Read the model definition and answer for the solid it produces. Units are mm, in the model's axes. A direction names the side the tool comes from. Coordinates: 2 decimals unless noted, no trailing zeros. Write each loop counter-clockwise with the first axis right and the second up, starting at its lowest first coordinate (ties: lowest second). Pieces come first, ordered by that corner, then holes.
(1) Section D-D on z = 32 is taken. Write down the section's boundary in (x, y), then the cut area to 3 significant figures.
(2) Section C-C on x = 30 is taken. Write down the section's boundary in (y, z), then the cut area to 3 significant figures.
(3) The mould has two halves that part along Z. Classify faces 4 (the cylindrical face through (55.07, 13.37, 24.68)), 5 (the flat face through (53, 0, 13)), 6 (the flat face through (21, 20, 10)): +Z half, -Z half, draft (parallel to the pull), parting line (faces both ways), or undercut.
(4) Given pin 1 (8 mm diameter, centred on x = 19, y = 22, fed in from +Z); pin 2 (10 mm diameter, centred on x = 36, z = 5.5, fed in from +Y) (3 decimals); pin 3 (5 mm diameter, centred on x = 51, z = 25, fed in from -Y); pin 4 (24 mm diameter, centred on y = 15, z = 32, fed in from -X), each flat-ended and moving along its own axis, determine where each tip first touches the part or whether it passes through.
(5) Section B-B on z = 8 is taken. Write down the section's boundary in (x, y).
(6) Section A-A on y = 15 is taken. Write down the section's boundary in (x, z), then the cut area to 3 significant figures.
(7) Which of the six approach directions +Z, -Z, +X, -X, +Y, -Y give full straight-line access (tool end or side, diameter ignored) to faces 1 (the cylindrical face through (17.47, 3.51, -1.48)), 2 (the flat face through (10, 19, 25)), 3 (the flat face through (7, 30, 13))?
(8) Find the intervals of material crossed by probe 1 along X at (y, z) = (28.5, 17); probe 2 along Y at (x, z) = (30, 6.5); probe 3 along X at (y, z) = (15, 0.75), in increasing order.
from build123d import *

# Parameters (mm, degrees)
F0_R     = 10
F1_DEPTH = 50
F2_R     = 10
F3_DEPTH = 40
F4_R     = 7.5
F5_DEPTH = 60.001
F6_R     = 17
F6_R_2   = 10
F7_DEPTH = 3


with BuildPart() as f1:
    # F0 (on Top) → F1 (new body)
    with BuildSketch(Plane.XY):
        with BuildLine():
            Line((43.2287565553, 0), (16.7712434447, 0))
            ThreePointArc((16.7712434447, 0), (30, -5), (43.2287565553, 0))
        make_face()
        Polygon((0, 30), (0, 0), (16.7712434447, 0), (43.2287565553, 0), (60, 0), (60, 30), (43.2287565553, 30), (16.7712434447, 30), align=None)
        with Locations((30, 15)):
            Circle(F0_R, mode=Mode.SUBTRACT)
        with BuildLine():
            ThreePointArc((43.2287565553, 30), (30, 35), (16.7712434447, 30))
            Line((16.7712434447, 30), (43.2287565553, 30))
        make_face()
    extrude(amount=F1_DEPTH)

    # F2 (on face) → F3 (cut)
    with BuildSketch(Plane.XY.offset(50)):
        with BuildLine():
            ThreePointArc((43.2287565553, 30), (37.0710678119, 33.7082869339), (30, 35))
            ThreePointArc((30, 35), (22.9289321881, 33.7082869339), (16.7712434447, 30))
            Line((16.7712434447, 30), (10, 30))
            Line((10, 30), (10, 0))
            Line((10, 0), (16.7712434447, 0))
            ThreePointArc((16.7712434447, 0), (22.9289321949, -3.7082869364), (30.0000000144, -5))
            ThreePointArc((30.0000000144, -5), (37.0710678186, -3.7082869313), (43.2287565553, 0))
            Line((43.2287565553, 0), (50, 0))
            Line((50, 0), (50, 30))
            Line((50, 30), (43.2287565553, 30))
        make_face()
        with Locations((30, 15)):
            Circle(F2_R, mode=Mode.SUBTRACT)
    extrude(amount=-F3_DEPTH, mode=Mode.SUBTRACT)

    # F4 (on face) → F5 (cut, through all)
    with BuildSketch(Plane.YZ.offset(60)):
        with BuildLine():
            Line((30, 50), (0, 50))
            Line((0, 50), (0, 35))
            ThreePointArc((0, 35), (15, 47.2970585408), (30, 35))
            Line((30, 35), (30, 50))
        make_face()
        with Locations((15, 32)):
            Circle(F4_R)
    extrude(amount=-F5_DEPTH, mode=Mode.SUBTRACT)

    # F6 (on face) → F7 (join)
    with BuildSketch(Plane(origin=(0, 0, 0), x_dir=(1, 0, 0), z_dir=(0, 0, -1))):
        with Locations((30, -15)):
            Circle(F6_R)
        with Locations((30, -15)):
            Circle(F6_R_2, mode=Mode.SUBTRACT)
    extrude(amount=F7_DEPTH)


solid = f1.part
Response:
1. outline: (0, 0) - (10, 0) - (10, 7.5) - (0, 7.5) - close; (0, 22.5) - (10, 22.5) - (10, 30) - (0, 30) - close; (50, 0) - (60, 0) - (60, 7.5) - (50, 7.5) - close; (50, 22.5) - (60, 22.5) - (60, 30) - (50, 30) - close
1. area: 300 mm2
2. outline: (-5, 0) - (-2, 0) - (-2, -3) - (5, -3) - (5, 10) - (-5, 10) - close; (25, -3) - (32, -3) - (32, 0) - (35, 0) - (35, 10) - (25, 10) - close
2. area: 242 mm2
3. face 4: undercut
3. face 5: draft
3. face 6: +Z half
4. pin 1: stops at z = 10
4. pin 2: stops at y = 34.975
4. pin 3: stops at y = 0
4. pin 4: stops at x = 0
5. outline: (0, 0) - (16.77, 0) arc R20 ccw to (43.23, 0) - (60, 0) - (60, 30) - (43.23, 30) arc R20 ccw to (16.77, 30) - (0, 30) - close; hole circle Ø20 at (30, 15)
6. outline: (0, 0) - (13, 0) - (13, -3) - (20, -3) - (20, 10) - (10, 10) - (10, 24.5) - (0, 24.5) - close; (0, 39.5) - (10, 39.5) - (10, 47.3) - (0, 47.3) - close; (40, -3) - (47, -3) - (47, 0) - (60, 0) - (60, 24.5) - (50, 24.5) - (50, 10) - (40, 10) - close; (50, 39.5) - (60, 39.5) - (60, 47.3) - (50, 47.3) - close
6. area: 888 mm2
7. face 1: -Z
7. face 2: +Z, +Y, -Y
7. face 3: +Z, -Z, -X, +Y
8. probe 1: x = 0 to 10, 50 to 60
8. probe 2: y = -5 to 5, 25 to 35
8. probe 3: x = 0 to 20, 40 to 60
